Model file for the job. Use its own axes, mm. Coordinates: 2 decimals unless noted, no trailing zeros. Write each loop counter-clockwise with the first axis right and the second up, starting at its lowest first coordinate (ties: lowest second). Pieces come first, ordered by that corner, then holes.
Q1. Drill centre lines: probe 1 along X at (y, z) = (1.85, -13); probe 2 along X at (y, z) = (2.45, -74). Where is each one in solid material? Low to high.
Q2. Band-saw the part on A-A, the plane y = 2.35. Write the cut outline in (x, z), plus the area to 3 significant figures.
Q3. Band-saw the part on B-B, the plane z = -278.5. Write the cut outline in (x, y), plus the area to 3 significant figures.
Q4. Pin check, flat tips, straight feed: P1, Ø1.5, axis at y = 3, z = -191, coming from the +X side; P2, Ø1.8, axis at y = 3.5, z = -21, coming from the -X side; P3, Ø1.5, axis at y = 4, z = -109.5, coming from the +X side. Stop position of each tip, or through.
Autodesk Inventor part; units mm, degrees
ref_plane "YZ Plane" through (0, 0, 0) normal (1, 0, 0) x (0, 1, 0)
ref_plane "XZ Plane" through (0, 0, 0) normal (0, 1, 0) x (-1, 0, 0)
ref_plane "XY Plane" through (0, 0, 0) normal (0, 0, 1) x (1, 0, 0)
sketch "Sketch1" plane through (0, 0, 0) normal (0, 1, 0) x (-1, 0, 0)
  line L0 (0, 0) -> (0, -312.648) construction
  line L1 (5, 0) -> (5, -312.648)
  line L2 (-5, -312.648) -> (-5, 0)
  arc A0 (5, 0) -> (-5, 0) centre (0, 0) ccw
  arc A1 (-5, -312.648) -> (5, -312.648) centre (0, -312.648) ccw
  circle A2 centre (0, 0) radius 1.65
  circle A3 centre (0, -312.648) radius 1.65
  circle A4 centre (0, -42.6) radius 1.65
  circle A5 centre (0, -254.274) radius 1.65
  arc A6 (5, -254.274) -> (5, -42.6) centre (-585.5917, -148.437) ccw
  arc A7 (-5, -254.274) -> (-5, -42.6) centre (-595.5917, -148.437) ccw
  circle A8 centre (7.5096, -100) radius 1.65
  point P0 (0, -156.324)
  dimension "d0" = 3.3
  dimension "d1" = 3.3
  dimension "d2" = 10
  dimension "d3" = 312.648
  dimension "d10" = 3.3
  dimension "d11" = 42.6
  dimension "d12" = 3.3
  dimension "d13" = 254.274
  dimension "d16" = 600
  dimension "d17" = 600
  dimension "d18" = 3.3
  dimension "d19" = 100
extrude "Extrusion1" add sketch "Sketch1" along normal blind 6 contours L1 A1 L2 A7 A0 | A6 L1
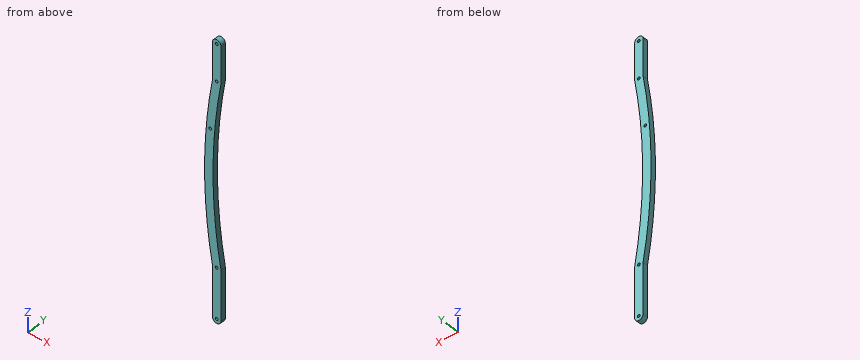
Answer sheet:
1. probe 1: x = -5 to 5
1. probe 2: x = -9.77 to 0.23
2. outline: (-5, -312.65) arc R5 ccw to (5, -312.65) - (5, -254.27) arc R600 cw to (5, -42.6) - (5, 0) arc R5 ccw to (-5, 0) - (-5, -42.6) arc R600 ccw to (-5, -254.27) - close; hole circle Ø3.3 at (-7.51, -100); hole circle Ø3.3 at (0, -312.65); hole circle Ø3.3 at (0, -254.27); hole circle Ø3.3 at (0, -42.6); hole circle Ø3.3 at (0, 0)
2. area: 3,160 mm2
3. outline: (-5, 0) - (5, 0) - (5, 6) - (-5, 6) - close
3. area: 60.0 mm2
4. P1: stops at x = -2.84
4. P2: stops at x = -5
4. P3: stops at x = -3.09
